Geometry check sheet. Reference: the model listing, model coordinates, mm. Face numbers are marked on the shaded views. A direction names the side the tool comes from. Coordinates: 2 decimals unless noted, no trailing zeros. Order: outer loops, then holes, each group sorted by start corner. A loop starts at its lowest first (then second) coordinate and runs counter-clockwise, first axis right, second up. Notation, with made-up numbers: (-28, 83) -> (27, 83) arc R26 ccw to (27, 108) -> close; hole circle Ø2 at (42, 36.25). An arc over 180 degrees is marked (long way). Answer in a Markdown table with one row per item. Add a question column.
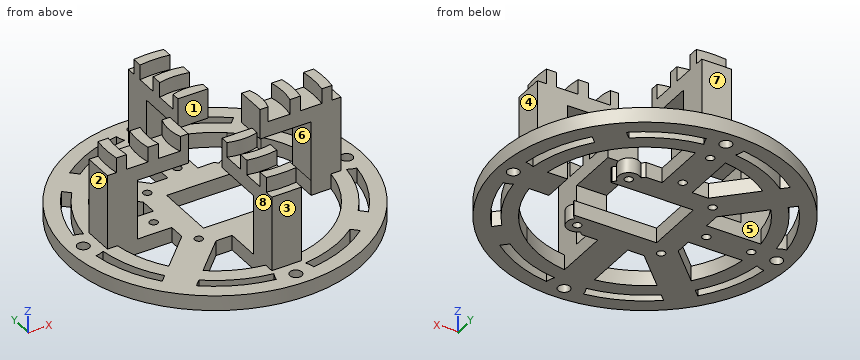
```python
from build123d import *

# Parameters (mm, degrees)
SKETCH1_R            = 49
BOSS_EXTRUDE1_DEPTH  = 5
CUT_EXTRUDE11_DEPTH  = 6
SKETCH24_R           = 1.35
CUT_EXTRUDE12_DEPTH  = 6
SKETCH25_R           = 2
CUT_EXTRUDE13_DEPTH  = 6
CIRPATTERN6_COUNT    = 4
SKETCH26_W           = 10
SKETCH26_H           = 10
BOSS_EXTRUDE23_DEPTH = 20
CIRPATTERN7_COUNT    = 4
SKETCH28_W           = 10
SKETCH28_H           = 27
BOSS_EXTRUDE25_DEPTH = 5
CIRPATTERN9_COUNT    = 4
BOSS_EXTRUDE26_DEPTH = 5
CIRPATTERN10_COUNT   = 4
SKETCH30_R           = 41
SKETCH30_R_2         = 36
BOSS_EXTRUDE27_DEPTH = 5
CUT_EXTRUDE14_DEPTH  = 5
SKETCH32_W           = 20
SKETCH32_H           = 20
SKETCH32_W_2         = 7.5
CUT_EXTRUDE15_DEPTH  = 5
SKETCH34_R           = 1.35
CUT_EXTRUDE16_DEPTH  = 5
CIRPATTERN11_COUNT   = 2
CIRPATTERN11_ANGLE   = 90


with BuildPart() as part:
    # Sketch1 → Boss-Extrude1 (new body)
    with BuildSketch(Plane.XY):
        Circle(SKETCH1_R)
    extrude(amount=BOSS_EXTRUDE1_DEPTH)

    # Sketch23 → Cut-Extrude11 (cut, through all)
    with BuildSketch(Plane.XY.offset(5)):
        with BuildLine():
            ThreePointArc((-40.313027208, 5), (-41.852174996, 5.829289504), (-43.56143445, 6.196888625))
            ThreePointArc((-43.56143445, 6.196888625), (-40.415985736, 17.393909768), (-34.446696938, 27.375629126))
            Line((-34.446696938, 27.375629126), (-17.5, 10.428932188))
            Line((-17.5, 10.428932188), (-17.5, 5))
            Line((-17.5, 5), (-40.313027208, 5))
        make_face()
        with BuildLine():
            ThreePointArc((-43.56143445, -6.196888625), (-41.852174996, -5.829289504), (-40.313027208, -5))
            Line((-40.313027208, -5), (-17.5, -5))
            Line((-17.5, -5), (-17.5, -10.428932188))
            Line((-17.5, -10.428932188), (-34.446696938, -27.375629126))
            ThreePointArc((-34.446696938, -27.375629126), (-40.415985736, -17.393909768), (-43.56143445, -6.196888625))
        make_face()
        with BuildLine():
            ThreePointArc((-5, -40.313027208), (-5.829289504, -41.852174996), (-6.196888625, -43.56143445))
            ThreePointArc((-6.196888625, -43.56143445), (-17.393909768, -40.415985736), (-27.375629126, -34.446696938))
            Line((-27.375629126, -34.446696938), (-10.428932188, -17.5))
            Line((-10.428932188, -17.5), (-5, -17.5))
            Line((-5, -17.5), (-5, -40.313027208))
        make_face()
        with BuildLine():
            ThreePointArc((6.196888625, -43.56143445), (5.829289504, -41.852174996), (5, -40.313027208))
            Line((5, -40.313027208), (5, -17.5))
            Line((5, -17.5), (10.428932188, -17.5))
            Line((10.428932188, -17.5), (27.375629126, -34.446696938))
            ThreePointArc((27.375629126, -34.446696938), (17.393909768, -40.415985736), (6.196888625, -43.56143445))
        make_face()
        with BuildLine():
            ThreePointArc((43.56143445, 6.196888625), (41.852174996, 5.829289504), (40.313027208, 5))
            Line((40.313027208, 5), (17.5, 5))
            Line((17.5, 5), (17.5, 10.428932188))
            Line((17.5, 10.428932188), (34.446696938, 27.375629126))
            ThreePointArc((34.446696938, 27.375629126), (40.415985736, 17.393909768), (43.56143445, 6.196888625))
        make_face()
        with BuildLine():
            Line((10.428932188, 17.5), (27.375629126, 34.446696938))
            ThreePointArc((27.375629126, 34.446696938), (17.393909768, 40.415985736), (6.196888625, 43.56143445))
            ThreePointArc((6.196888625, 43.56143445), (5.829289504, 41.852174996), (5, 40.313027208))
            Line((5, 40.313027208), (5, 17.5))
            Line((5, 17.5), (10.428932188, 17.5))
        make_face()
        with BuildLine():
            ThreePointArc((-6.196888625, 43.56143445), (-5.829289504, 41.852174996), (-5, 40.313027208))
            Line((-5, 40.313027208), (-5, 17.5))
            Line((-5, 17.5), (-10.428932188, 17.5))
            Line((-10.428932188, 17.5), (-27.375629126, 34.446696938))
            ThreePointArc((-27.375629126, 34.446696938), (-17.393909768, 40.415985736), (-6.196888625, 43.56143445))
        make_face()
        with BuildLine():
            Line((17.5, -10.428932188), (34.446696938, -27.375629126))
            ThreePointArc((34.446696938, -27.375629126), (40.415985736, -17.393909768), (43.56143445, -6.196888625))
            ThreePointArc((43.56143445, -6.196888625), (41.852174996, -5.829289504), (40.313027208, -5))
            Line((40.313027208, -5), (17.5, -5))
            Line((17.5, -5), (17.5, -10.428932188))
        make_face()
    extrude(amount=-CUT_EXTRUDE11_DEPTH, mode=Mode.SUBTRACT)

    # Sketch24 → Cut-Extrude12 (cut, through all)
    with BuildSketch(Plane.XY.offset(5)):
        with Locations((-14, 14)):
            Circle(SKETCH24_R)
        with Locations((14, 14)):
            Circle(SKETCH24_R)
        with Locations((14, -14)):
            Circle(SKETCH24_R)
        with Locations((-14, -14)):
            Circle(SKETCH24_R)
    extrude(amount=-CUT_EXTRUDE12_DEPTH, mode=Mode.SUBTRACT)

    # Sketch25 → Cut-Extrude13 (cut, through all)
    with BuildSketch(Plane.XY.offset(5)):
        with Locations((0, 44)):
            Circle(SKETCH25_R)
    cut_extrude13 = extrude(amount=-CUT_EXTRUDE13_DEPTH, mode=Mode.SUBTRACT)

    # CirPattern6: Cut-Extrude13 ×4 about axis
    cirpattern6_axis = Axis((0, 0, 0), (0, 0, 1))
    for i in range(1, CIRPATTERN6_COUNT):
        add(cut_extrude13.rotate(cirpattern6_axis, i * 360 / CIRPATTERN6_COUNT), mode=Mode.SUBTRACT)

    # Sketch26 → Boss-Extrude23 (add)
    with BuildSketch(Plane.XY.offset(5)):
        with Locations((0, 34)):
            Rectangle(SKETCH26_W, SKETCH26_H)
    boss_extrude23 = extrude(amount=BOSS_EXTRUDE23_DEPTH)

    # CirPattern7: Boss-Extrude23 ×4 about axis
    cirpattern7_axis = Axis((0, 0, 0), (0, 0, 1))
    for i in range(1, CIRPATTERN7_COUNT):
        add(boss_extrude23.rotate(cirpattern7_axis, i * 360 / CIRPATTERN7_COUNT))

    # Sketch28 → Boss-Extrude25 (add)
    with BuildSketch(Plane.XY.offset(25)):
        with Locations((0, 25.5)):
            Rectangle(SKETCH28_W, SKETCH28_H)
    boss_extrude25 = extrude(amount=BOSS_EXTRUDE25_DEPTH)

    # CirPattern9: Boss-Extrude25 ×4 about axis
    cirpattern9_axis = Axis((0, 0, 0), (0, 0, 1))
    for i in range(1, CIRPATTERN9_COUNT):
        add(boss_extrude25.rotate(cirpattern9_axis, i * 360 / CIRPATTERN9_COUNT))

    # Sketch29 → Boss-Extrude26 (add)
    with BuildSketch(Plane.XY.offset(30)):
        with BuildLine():
            ThreePointArc((-5, 32.619012861), (0, 33), (5, 32.619012861))
            Line((5, 32.619012861), (5, 36.024670713))
            ThreePointArc((5, 36.024670713), (0, 36.37), (-5, 36.024670713))
            Line((-5, 36.024670713), (-5, 32.619012861))
        make_face()
        with BuildLine():
            ThreePointArc((-5, 21.937410968), (0, 22.5), (5, 21.937410968))
            Line((5, 21.937410968), (5, 25.463748742))
            ThreePointArc((5, 25.463748742), (0, 25.95), (-5, 25.463748742))
            Line((-5, 25.463748742), (-5, 21.937410968))
        make_face()
        with BuildLine():
            Line((-5, 12), (5, 12))
            Line((5, 12), (5, 14.671400751))
            ThreePointArc((5, 14.671400751), (0, 15.5), (-5, 14.671400751))
            Line((-5, 14.671400751), (-5, 12))
        make_face()
    boss_extrude26 = extrude(amount=BOSS_EXTRUDE26_DEPTH)

    # CirPattern10: Boss-Extrude26 ×4 about axis
    cirpattern10_axis = Axis((0, 0, 0), (0, 0, 1))
    for i in range(1, CIRPATTERN10_COUNT):
        add(boss_extrude26.rotate(cirpattern10_axis, i * 360 / CIRPATTERN10_COUNT))

    # Sketch30 → Boss-Extrude27 (add)
    with BuildSketch(Plane(origin=(0, 0, 0), x_dir=(-1, 0, 0), z_dir=(0, 0, -1))):
        Circle(SKETCH30_R)
        Circle(SKETCH30_R_2, mode=Mode.SUBTRACT)
    extrude(amount=-BOSS_EXTRUDE27_DEPTH)

    # Sketch31 → Cut-Extrude14 (cut)
    with BuildSketch(Plane(origin=(0, 0, 0), x_dir=(-1, 0, 0), z_dir=(0, 0, -1))):
        with BuildLine():
            Line((-5, 35.65108694), (-5, 17.5))
            Line((-5, 17.5), (-10.428932188, 17.5))
            Line((-10.428932188, 17.5), (-11.489847469, 16.43908472))
            ThreePointArc((-11.489847469, 16.43908472), (-16.474873734, 16.474873734), (-16.43908472, 11.489847469))
            Line((-16.43908472, 11.489847469), (-17.5, 10.428932188))
            Line((-17.5, 10.428932188), (-17.5, -10.428932188))
            Line((-17.5, -10.428932188), (-16.449876269, -11.500378775))
            ThreePointArc((-16.449876269, -11.500378775), (-16.474873734, -16.474873734), (-11.500378775, -16.449876269))
            Line((-11.500378775, -16.449876269), (-10.428932188, -17.5))
            Line((-10.428932188, -17.5), (-5, -17.5))
            Line((-5, -17.5), (-5, -35.65108694))
            ThreePointArc((-5, -35.65108694), (-25.455844123, -25.455844123), (-35.65108694, -5))
            Line((-35.65108694, -5), (-29.00108694, -5))
            Line((-29.00108694, -5), (-29.00108694, 5))
            Line((-29.00108694, 5), (-35.65108694, 5))
            ThreePointArc((-35.65108694, 5), (-25.455844123, 25.455844123), (-5, 35.65108694))
        make_face()
    extrude(amount=-CUT_EXTRUDE14_DEPTH, mode=Mode.SUBTRACT)

    # Sketch32 → Cut-Extrude15 (cut)
    with BuildSketch(Plane(origin=(0, 0, 0), x_dir=(-1, 0, 0), z_dir=(0, 0, -1))):
        Rectangle(SKETCH32_W, SKETCH32_H)
        with Locations((-13.75, 0)):
            Rectangle(SKETCH32_W_2, SKETCH32_H)
    extrude(amount=-CUT_EXTRUDE15_DEPTH, mode=Mode.SUBTRACT)

    # Sketch34 → Cut-Extrude16 (cut)
    with BuildSketch(Plane(origin=(0, 0, 0), x_dir=(-1, 0, 0), z_dir=(0, 0, -1))):
        with Locations((0, 20.5)):
            Circle(SKETCH34_R)
        with Locations((0, 35.5)):
            Circle(SKETCH34_R)
    cut_extrude16 = extrude(amount=-CUT_EXTRUDE16_DEPTH, mode=Mode.SUBTRACT)

    # CirPattern11: Cut-Extrude16 ×2 about axis
    cirpattern11_axis = Axis((0, 0, 0), (0, 0, 1))
    for i in range(1, CIRPATTERN11_COUNT):
        add(cut_extrude16.rotate(cirpattern11_axis, i * CIRPATTERN11_ANGLE / (CIRPATTERN11_COUNT - 1)), mode=Mode.SUBTRACT)


solid = part.part
```
(1) Access from +Z, -Z, +X, -X, +Y, -Y to the whole of each face (thin tool, end or side, straight path). Record for the marked faces 1, 2, 3, 4 and 5.
(2) Go/stop test with flat-tipped pins: P1, Ø4, axis at x = 35, z = 5, coming from the -Y side; P2, Ø8.5, axis at x = -30, y = -2, coming from the +Z side; P3, Ø5, axis at x = 20.5, y = 2, coming from the -Z side; P4, Ø2, axis at y = -26, z = 25.5, coming from the -X side. Record where each tip stops, or that it passes through.
(3) Mould release check, pull along Y, two halves, no side actions. Record for the marked faces 6, 7 and 8: +Y half, -Y half, draft (parallel to the pull), parting line (faces both ways), or undercut.
(4) Scan lines: line 1 along Y through (x, z) = (0, 2.7); line 2 along Y through (x, z) = (2, 11.5); line 3 along Z through (x, y) = (3.5, -25). Record each from-to range of solid material in increasing order.
(5) Cross-section at B-B (y = 20.5). Give the number of separate pieces and of enclosed holes in the cut face, plus the area to 3 significant figures.
(6) Cross-section at A-A (z = 22). Enter the section's corners in (x, y).
Checks:
| question | item | result |
|---|---|---|
| 1 | face 1 | +Z, +X, -X |
| 1 | face 2 | +Z, -X, +Y, -Y |
| 1 | face 3 | +Z, +X, -X, -Y |
| 1 | face 4 | +Z, +X, +Y, -Y |
| 1 | face 5 | +Z |
| 2 | P1 | y = -36.22 |
| 2 | P2 | z = 35 |
| 2 | P3 | z = 25 |
| 2 | P4 | x = -5 |
| 3 | face 6 | draft |
| 3 | face 7 | +Y half |
| 3 | face 8 | undercut |
| 4 | line 1 | -49 to -46, -42 to -10, 10 to 19.15, 21.85 to 34.15, 36.85 to 42, 46 to 49 |
| 4 | line 2 | -39 to -29, 29 to 39 |
| 4 | line 3 | 0 to 5, 25 to 35 |
| 5 | separate pieces | 8 |
| 5 | enclosed holes | 0 |
| 5 | area | 272 mm² |
| 6 | outline | (-39, -5) -> (-29, -5) -> (-29, 5) -> (-39, 5) -> close; (-5, -39) -> (5, -39) -> (5, -29) -> (-5, -29) -> close; (-5, 29) -> (5, 29) -> (5, 39) -> (-5, 39) -> close; (29, -5) -> (39, -5) -> (39, 5) -> (29, 5) -> close |
